Autodesk Inventor part; units mm, degrees
ref_plane "YZ Plane" through (0, 0, 0) normal (1, 0, 0) x (0, 1, 0)
ref_plane "XZ Plane" through (0, 0, 0) normal (0, 1, 0) x (-1, 0, 0)
ref_plane "XY Plane" through (0, 0, 0) normal (0, 0, 1) x (1, 0, 0)
sketch "Sketch2" plane through (0, 0, 0) normal (0, 1, 0) x (-1, 0, 0)
  line L0 (0, 0) -> (2.85, 0)
  line L1 (2.85, 0) -> (2.85, -1.65)
  line L2 (2.85, -1.65) -> (1.25, -1.65)
  line L3 (1.25, -1.65) -> (1.25, -6.65)
  line L4 (1.25, -6.65) -> (0, -6.65)
  line L5 (0, 0) -> (0, -6.65)
  dimension "d9" = 2.85
  dimension "d10" = 1.65
  dimension "d12" = 5
  dimension "d19" = 2.5
revolve "Revolution1" add sketch "Sketch2" angle 360 about axis through (0, 0, 0) along (0, 0, -1)
fillet "Fillet1" radius 1.5 1 edges at (2.85, 0, 0)
chamfer "Chamfer1" distance 0.2 angle 45 1 edges at (1.25, 0, -6.65)
thread "Thread1"
sketch "Sketch4" plane through (0, 0, 0) normal (0, 0, 1) x (1, 0, 0)
  line L0 (0, 0.866) -> (0.75, 0.433)
  line L1 (0.75, 0.433) -> (0.75, -0.433)
  line L2 (0.75, -0.433) -> (0, -0.866)
  line L3 (0, -0.866) -> (-0.75, -0.433)
  line L4 (-0.75, -0.433) -> (-0.75, 0.433)
  line L5 (-0.75, 0.433) -> (0, 0.866)
  circle A0 centre (0, 0) radius 1.05
  point P0 (0, 0)
  dimension "d22" = 1.5
  dimension "d30" = 0.433
extrude "Extrusion2" cut sketch "Sketch4" against normal blind 1 contours L0 L1 L2 L3 L4 L5
chamfer "Chamfer2" distance 0.1 angle 45 12 edges at (-0.75, 0, 0) (-0.375, 0.6495, 0) (0.375, 0.6495, 0) (0.75, 0, 0) (0.375, -0.6495, 0) (-0.375, -0.6495, 0) (-0.375, 0.6495, -1) (-0.75, 0, -1) (-0.375, -0.6495, -1) (0.375, -0.6495, -1) (0.75, 0, -1) (0.375, 0.6495, -1)
properties part number "rapoukHexagonScrewM2,5v0" material "Steel, Carbon"
The listing builds one solid part. Answer for the finished solid, in the listing's coordinates (mm). A direction names the side the tool comes from. Give positions to 0.01 mm unless a question says otherwise; leave off trailing zeros. Write each loop counter-clockwise with the first axis right and the second up, starting at its lowest first coordinate (ties: lowest second). Pieces come first, ordered by that corner, then holes. Notation, with made-up numbers: (39, 13) - (48, 13) arc R20 cw to (48, 40) - close; hole circle Ø2 at (18, 26.25). An arc over 180 degrees is marked (long way). Use a Markdown table: item, result.
1. Find the intervals of material crossed by probe 1 along Z at (x, y) = (-0.1, -1.4); probe 2 along Z at (x, y) = (1.7, 1.7); probe 3 along Y at (x, z) = (-2.25, -1), in increasing order. Write a range as from..to.
Values follow:
| item | result |
|---|---|
| probe 1 | z = -1.65..0 |
| probe 2 | z = -1.65..-0.43 |
| probe 3 | y = -1.61..1.61 |
2. Section A-A on z = -5.5 is taken. Write down the section's boundary in (x, y), plus the area to 3 significant figures.
Values follow:
| item | result |
|---|---|
| outline | circle Ø2.5 at (0, 0) |
| area | 4.91 mm² |
3. Each of these flat-tipped pins is pushed along its axis until it touches: P1, Ø1, axis at x = 1.5, y = -1.5, coming from the +Z side; P2, Ø0.9, axis at y = 0, z = -0.5, coming from the -X side; P3, Ø2, axis at y = 1.5, z = -1.5, coming from the -X side. Where does it stop, or does it pass through?
Values follow:
| item | result |
|---|---|
| P1 | stops at z = -0.02 |
| P2 | stops at x = -2.75 |
| P3 | stops at x = -2.81 |
4. A tool of negligible diameter and unlimited length cuts with its end or side. For faces 1 (the flat face through (-1, 0, 0)), 2 (the flat face through (-1, -1, -1.65)), 3 (the flat face through (0, 0, -1)), from which of +Z, -Z, +X, -X, +Y, -Y can it reach the whole face along a straight path? Write none if from no direction.
Values follow:
| item | result |
|---|---|
| face 1 | +Z, +X, -X, +Y, -Y |
| face 2 | -Z |
| face 3 | +Z |
